Source: CAD feature listing. Evaluate the final solid. Frame: model axes, mm. A direction names the side the tool comes from. Round coordinates to 2 decimals unless told otherwise and drop trailing zeros. Write each loop counter-clockwise with the first axis right and the second up, starting at its lowest first coordinate (ties: lowest second). Pieces come first, ordered by that corner, then holes. Notation, with made-up numbers: (60, 1.5) -> (105, 1.5) arc R27 ccw to (105, 18.5) -> close; hole circle Ø2 at (83, 37.5). An arc over 180 degrees is marked (long way). Return JSON: item names as keys, results as strings. Group by question number.
from build123d import *

# Parameters (mm, degrees)
EXTRUDE_1_DEPTH     = 21
EXTRUDE_2_DEPTH     = 3
SKETCH_4_W          = 27
SKETCH_4_H          = 125.4
CUT_EXTRUDE_1_DEPTH = 16.5
CUT_EXTRUDE_3_DEPTH = 32
SKETCH_6_W          = 32
SKETCH_6_H          = 32
CUT_EXTRUDE_4_DEPTH = 16.5
FILLET_1_R          = 3
SWEEP_START         = 3
SWEEP_3_DEPTH       = 3
SWEEP_START_2       = 9
SWEEP_3_2_DEPTH     = 3
SWEEP_START_3       = 15
SWEEP_3_3_DEPTH     = 3


# Read off the part's stored shape, not the designer's step: Вырез-По траектории3
with BuildPart() as part:
    # Эскиз1 → Бобышка-Вытянуть1 (new body)
    with BuildSketch(Plane(origin=(0, 0, 0), x_dir=(0, 0, -1), z_dir=(1, 0, 0))):
        with BuildLine():
            Line((-56, -42), (-34.436750731, -25.75092618))
            ThreePointArc((-34.436750731, -25.75092618), (0, 43), (34.436750731, -25.75092618))
            Line((34.436750731, -25.75092618), (56, -42))
            Line((56, -42), (56, -166))
            Line((56, -166), (102, -131.336513695))
            Line((102, -131.336513695), (102, 0))
            ThreePointArc((102, 0), (0, 102), (-102, 0))
            Line((-102, 0), (-102, -131.336513695))
            Line((-102, -131.336513695), (-56, -166))
            Line((-56, -166), (-56, -42))
        make_face()
    extrude(amount=EXTRUDE_1_DEPTH)

    # Эскиз3 → Бобышка-Вытянуть2 (add)
    with BuildSketch(Plane(origin=(21, 0, 0), x_dir=(0, 0, -1), z_dir=(1, 0, 0))):
        with BuildLine():
            Line((-57, -41.501418392), (-35.82524401, -25.545095256))
            ThreePointArc((-35.82524401, -25.545095256), (0, 44), (35.82524401, -25.545095256))
            Line((35.82524401, -25.545095256), (57, -41.501418392))
            Line((57, -41.501418392), (57, -164))
            Line((57, -164), (101, -130.843621795))
            Line((101, -130.843621795), (101, 0))
            ThreePointArc((101, 0), (0, 101), (-101, 0))
            Line((-101, 0), (-101, -130.843621795))
            Line((-101, -130.843621795), (-57, -164))
            Line((-57, -164), (-57, -41.501418392))
        make_face()
    extrude(amount=EXTRUDE_2_DEPTH)

    # Эскиз4 → Вырез-Вытянуть1 (cut)
    with BuildSketch(Plane.ZY):
        with Locations((-79.5, -62.7)):
            Rectangle(SKETCH_4_W, SKETCH_4_H)
    extrude(amount=-CUT_EXTRUDE_1_DEPTH, mode=Mode.SUBTRACT)

    # Sketch 1 2 → Вырез-Вытянуть3 (cut)
    with BuildSketch(Plane(origin=(0, 0, 95.5), x_dir=(0.400818834019707, -0.9161573349021895, 0), z_dir=(0, 0, 1))):
        Polygon((0, 0), (29.317034717, -12.826202689), (34.928498393, 0), (6.613510761, 15.116596026), align=None)
    extrude(amount=-CUT_EXTRUDE_3_DEPTH, mode=Mode.SUBTRACT)

    # Эскиз6 → Вырез-Вытянуть4 (cut)
    with BuildSketch(Plane.ZY):
        with Locations((79.5, -63)):
            Rectangle(SKETCH_6_W, SKETCH_6_H)
    extrude(amount=-CUT_EXTRUDE_4_DEPTH, mode=Mode.SUBTRACT)

    # Скругление1
    fillet_1_edges = [part.edges().sort_by_distance(p)[0] for p in [
        (8.25, -125.4, -66),
        (8.25, -125.4, -93),
        (8.25, 0, -66),
        (8.25, 0, -93),
        (8.25, -79, 95.5),
        (8.25, -79, 63.5),
        (8.25, -47, 95.5),
        (8.25, -47, 63.5),
        (7, -32, 63.5),
        (7, -32, 95.5),
        (8.25, 0, 63.5),
        (8.25, 0, 95.5),
    ]]
    fillet(fillet_1_edges, radius=FILLET_1_R)

    # Вырез-По траектории3 outline → Вырез-По траектории3 (cut)
    with BuildSketch(Plane.YZ.offset(SWEEP_START)):
        with BuildLine():
            Line((-25.153803165, 38.62926215), (-40.504255176, 59))
            Line((-40.504255176, 59), (-163.73933785, 59))
            Line((-163.73933785, 59), (-166, 56))
            Line((-166, 56), (-42, 56))
            Line((-42, 56), (-25.75092618, 34.436750731))
            ThreePointArc((-25.75092618, 34.436750731), (43, 0), (-25.75092618, -34.436750731))
            Line((-25.75092618, -34.436750731), (-42, -56))
            Line((-42, -56), (-166, -56))
            Line((-166, -56), (-163.73933785, -59))
            Line((-163.73933785, -59), (-40.504255176, -59))
            Line((-40.504255176, -59), (-25.153803165, -38.62926215))
            ThreePointArc((-25.153803165, -38.62926215), (46.097003242, 0), (-25.153803165, 38.62926215))
        make_face()
    extrude(amount=SWEEP_3_DEPTH, mode=Mode.SUBTRACT)

    # Sweep 3 2 outline → Sweep 3 2 (cut)
    with BuildSketch(Plane.YZ.offset(SWEEP_START_2)):
        with BuildLine():
            Line((-25.153803165, 38.62926215), (-40.504255176, 59))
            Line((-40.504255176, 59), (-163.73933785, 59))
            Line((-163.73933785, 59), (-166, 56))
            Line((-166, 56), (-42, 56))
            Line((-42, 56), (-25.75092618, 34.436750731))
            ThreePointArc((-25.75092618, 34.436750731), (43, 0), (-25.75092618, -34.436750731))
            Line((-25.75092618, -34.436750731), (-42, -56))
            Line((-42, -56), (-166, -56))
            Line((-166, -56), (-163.73933785, -59))
            Line((-163.73933785, -59), (-40.504255176, -59))
            Line((-40.504255176, -59), (-25.153803165, -38.62926215))
            ThreePointArc((-25.153803165, -38.62926215), (46.097003242, 0), (-25.153803165, 38.62926215))
        make_face()
    extrude(amount=SWEEP_3_2_DEPTH, mode=Mode.SUBTRACT)

    # Sweep 3 3 outline → Sweep 3 3 (cut)
    with BuildSketch(Plane.YZ.offset(SWEEP_START_3)):
        with BuildLine():
            Line((-25.153803165, 38.62926215), (-40.504255176, 59))
            Line((-40.504255176, 59), (-163.73933785, 59))
            Line((-163.73933785, 59), (-166, 56))
            Line((-166, 56), (-42, 56))
            Line((-42, 56), (-25.75092618, 34.436750731))
            ThreePointArc((-25.75092618, 34.436750731), (43, 0), (-25.75092618, -34.436750731))
            Line((-25.75092618, -34.436750731), (-42, -56))
            Line((-42, -56), (-166, -56))
            Line((-166, -56), (-163.73933785, -59))
            Line((-163.73933785, -59), (-40.504255176, -59))
            Line((-40.504255176, -59), (-25.153803165, -38.62926215))
            ThreePointArc((-25.153803165, -38.62926215), (46.097003242, 0), (-25.153803165, 38.62926215))
        make_face()
    extrude(amount=SWEEP_3_3_DEPTH, mode=Mode.SUBTRACT)


solid = part.part
Item 1: Cut plane B-B on z = 81. Output: boundary loops of the cut face in (x, y), and give its area (3 significant figures).
Item 2: Cut plane A-A on z = -13.5. Output: boundary loops of the cut face in (x, y), and give its area (3 significant figures).
Item 3: Material intervals for probe 1 along X at (y, z) = (-18.5, -42); probe 2 along Z at (x, y) = (4.25, -50); probe 3 along Z at (x, y) = (22.75, -57.5), sorted ascending.
Item 4: First-contact query: pin 1 Ø10 at (x, z) = (8.5, 7.5) entering from +Y; pin 2 Ø8 at (x, z) = (5.5, 21.5) entering from -Y; pin 3 Ø3 at (x, y) = (12.5, 50.5) entering from -Z. Flat tips, straight axial feed; report the tip coordinate or a pass-through.
Item 5: Pull-direction query (Z, two-part tool) for faces 4 (the flat face through (8, -47, 79)), 5 (the flat face through (0, -12, 46)), 6 (the flat face through (10.35, -148.91, -78.68)); classes: +Z half, -Z half, draft (parallel to the pull), parting line (faces both ways), or undercut.
Item 6: Set-up query: faces 1 (the flat face through (7, -32, 80)), 2 (the flat face through (4.48, -32.94, -48.96)), 3 (the flat face through (19.48, -33.99, 45.37)). Return all of +Z, -Z, +X, -X, +Y, -Y with unobstructed straight access to the full face (end or side cutting, diameter ignored); none if empty.
Here are the results:
{
 "1": {"outline": "(0, -147.16) -> (21, -147.16) -> (21, -145.91) -> (24, -145.91) -> (24, 60.33) -> (21, 60.33) -> (21, 61.99) -> (0, 61.99) -> (0, 0) -> (16.5, 0) -> (14, -32) -> (0, -32) -> (0, -47) -> (16.5, -47) -> (16.5, -79) -> (0, -79) -> close", "area": "3,990 mm^2"},
 "2": {"outline": "(0, 40.83) -> (3, 40.83) -> (3, 44.08) -> (6, 44.08) -> (6, 40.83) -> (9, 40.83) -> (9, 44.08) -> (12, 44.08) -> (12, 40.83) -> (15, 40.83) -> (15, 44.08) -> (18, 44.08) -> (18, 40.83) -> (21, 40.83) -> (21, 41.88) -> (24, 41.88) -> (24, 100.09) -> (21, 100.09) -> (21, 101.1) -> (0, 101.1) -> close", "area": "1,410 mm^2"},
 "3": {"probe 1": "x = 0 to 3, 6 to 9, 12 to 15, 18 to 24", "probe 2": "z = -102 to -93, -66 to -59, 59 to 63.5, 95.5 to 102", "probe 3": "z = -101 to -57, 57 to 101"},
 "4": {"pin 1": "stops at y = 101.97", "pin 2": "stops at y = 34.65", "pin 3": "stops at z = -89.46"},
 "5": {"face 4": "undercut", "face 5": "draft", "face 6": "-Z half"},
 "6": {"face 1": "-X", "face 2": "-Y", "face 3": "+X, -X, -Y"}
}
